Verification items for the finished model (mm, model axes). A direction names the side the tool comes from. Coordinates: 2 decimals unless noted, no trailing zeros. Write each loop counter-clockwise with the first axis right and the second up, starting at its lowest first coordinate (ties: lowest second). Pieces come first, ordered by that corner, then holes. Notation, with made-up numbers: (47, 57.25) -> (68, 57.25) arc R35 ccw to (68, 91.25) -> close; hole circle Ø7 at (54.25, 71). An arc over 180 degrees is marked (long way). Write each question's results on one line, items separated by ' | '. Start each with the question number.
from build123d import *

# Parameters (mm, degrees)
CROQUIS1_R              = 10
SALIENTE_EXTRUIR1_DEPTH = 2
CROQUIS2_R              = 5
SALIENTE_EXTRUIR2_DEPTH = 10
CORTAR_EXTRUIR1_DEPTH   = 8
SALIENTE_EXTRUIR3_START = 10
CROQUIS4_R              = 5
SALIENTE_EXTRUIR3_DEPTH = 10
REDONDEO1_R             = 3
CORTAR_EXTRUIR2_DEPTH   = 9


with BuildPart() as part:
    # Croquis1 → Saliente-Extruir1 (new, symmetric)
    with BuildSketch(Plane(origin=(0, 0, 0), x_dir=(1, 0, 0), z_dir=(0, 1, 0))):
        with Locations(Location((0, 0, 0), (0, 0, 270))):
            Circle(CROQUIS1_R)
    extrude(amount=SALIENTE_EXTRUIR1_DEPTH, both=True)

    # Croquis2 → Saliente-Extruir2 (add)
    with BuildSketch(Plane(origin=(0, 2, 0), x_dir=(1, 0, 0), z_dir=(0, 1, 0))):
        with Locations(Location((0, 0, 0), (0, 0, 270))):
            Circle(CROQUIS2_R)
    extrude(amount=SALIENTE_EXTRUIR2_DEPTH)

    # Croquis3 → Cortar-Extruir1 (cut)
    with BuildSketch(Plane(origin=(0, 12, 0), x_dir=(1, 0, 0), z_dir=(0, 1, 0))):
        with BuildLine():
            Line((-2.872281323, 2), (2.872281323, 2))
            ThreePointArc((2.872281323, 2), (0, -3.5), (-2.872281323, 2))
        make_face()
    extrude(amount=-CORTAR_EXTRUIR1_DEPTH, mode=Mode.SUBTRACT)

    # Croquis4 → Saliente-Extruir3 (add)
    with BuildSketch(Plane(origin=(0, -2, 0), x_dir=(-1, 0, 0), z_dir=(0, -1, 0)).offset(SALIENTE_EXTRUIR3_START)):
        with Locations(Location((0, 0, 0), (0, 0, 270))):
            Circle(CROQUIS4_R)
    extrude(amount=-SALIENTE_EXTRUIR3_DEPTH)

    # Redondeo1
    redondeo1_edges = [part.edges().sort_by_distance(p)[0] for p in [
        (0, -2, -5),
        (0, 2, -5),
    ]]
    fillet(redondeo1_edges, radius=REDONDEO1_R)

    # Croquis5 → Cortar-Extruir2 (cut)
    with BuildSketch(Plane.XZ.offset(12)):
        with BuildLine():
            Line((-2.1914607, 2.4), (2.1914607, 2.4))
            ThreePointArc((2.1914607, 2.4), (3.25, 0), (2.1914607, -2.4))
            Line((2.1914607, -2.4), (-2.1914607, -2.4))
            ThreePointArc((-2.1914607, -2.4), (-3.25, 0), (-2.1914607, 2.4))
        make_face()
    extrude(amount=-CORTAR_EXTRUIR2_DEPTH, mode=Mode.SUBTRACT)


solid = part.part
1. Material ranges on probe 1 along X at (y, z) = (10, 0); probe 2 along Y at (x, z) = (3.75, 8.5); probe 3 along Y at (x, z) = (3, -0.5), recorded low to high. Write a range as from..to.
2. Depth check by flat-ended pin: pin 1 Ø1.5 at (y, z) = (7.5, -3.5) entering from -X; pin 2 Ø3 at (x, z) = (-5, 5) entering from -Y; pin 3 Ø8 at (x, y) = (-7, -5) entering from +Z. Enter the tip coordinate at first touch or a pass-through.
3. Mould release check, pull along X, two halves, no side actions. Record for faces 4 (the cylindrical face through (0.1, 8.1, 3.5)), 5 (the cylindrical face through (-9.76, 0.03, -2.17)), 6 (the flat face through (8.2, 2, 0)): +X half, -X half, draft (parallel to the pull), parting line (faces both ways), or undercut.
4. Tool access check on faces 1 (the flat face through (0, -12, 3)), 2 (the cylindrical face through (-4.88, 8.45, -1.08)), 3 (the flat face through (0, -8, -2.4)). Record the directions out of +Z, -Z, +X, -X, +Y, -Y that give a thin tool (end or side, any length) a straight path to the whole face; none if there is none.
5. Sectioned sample at C-C on z = 0. Record the cut outline in (x, y).
6. Sectioned sample at B-B on y = 7. Record the cut outline in (x, z).
7. Sectioned sample at A-A on x = 0. Record the cut outline in (y, z), plus the area to 3 significant figures.
8. Sectioned sample at D-D on y = -0.5. Record the cut outline in (x, z).
Computed values:
1) probe 1: x = -5..-3.5, 3.5..5 | probe 2: y = -2..2 | probe 3: y = -3..4
2) pin 1: stops at x = -4.18 | pin 2: stops at y = -3.24 | pin 3: stops at z = 9
3) face 4: undercut | face 5: parting line | face 6: draft
4) face 1: +Z, -Z, +X, -X, -Y | face 2: +Y | face 3: -Y
5) outline: (-10, -2) -> (-8, -2) arc R3 cw to (-5, -5) -> (-5, -12) -> (-3.25, -12) -> (-3.25, -3) -> (3.25, -3) -> (3.25, -12) -> (5, -12) -> (5, -5) arc R3 cw to (8, -2) -> (10, -2) -> (10, 2) -> (8, 2) arc R3 cw to (5, 5) -> (5, 12) -> (3.5, 12) -> (3.5, 4) -> (-3.5, 4) -> (-3.5, 12) -> (-5, 12) -> (-5, 5) arc R3 cw to (-8, 2) -> (-10, 2) -> close
6) outline: circle Ø10 at (0, 0); hole (-2.87, -2) -> (2.87, -2) arc R3.5 ccw (long way) to start
7) outline: (-12, -5) -> (-5, -5) arc R3 cw to (-2, -8) -> (-2, -10) -> (2, -10) -> (2, -8) arc R3 cw to (5, -5) -> (12, -5) -> (12, -2) -> (4, -2) -> (4, 3.5) -> (12, 3.5) -> (12, 5) -> (5, 5) arc R3 cw to (2, 8) -> (2, 10) -> (-2, 10) -> (-2, 8) arc R3 cw to (-5, 5) -> (-12, 5) -> (-12, 2.4) -> (-3, 2.4) -> (-3, -2.4) -> (-12, -2.4) -> close | area: 201 mm^2
8) outline: circle Ø20 at (0, 0)
